```python
from build123d import *

# Parameters (mm, degrees)
BOSS_EXTRUDE1_DEPTH = 14
SKETCH2_R           = 2
CUT_EXTRUDE1_DEPTH  = 52.751714947


with BuildPart() as part:
    # Sketch1 → Boss-Extrude1 (new body)
    with BuildSketch(Plane.XY):
        with BuildLine():
            Line((0, 0), (42, 0))
            Line((42, 0), (42, 6))
            Line((42, 6), (30, 6))
            Line((30, 6), (30, 32.8))
            Line((30, 32.8), (22.249007882, 32.8))
            Line((22.249007882, 32.8), (22.249007882, 23.8))
            ThreePointArc((22.249007882, 23.8), (21, 15.999997414), (19.750992118, 23.8))
            Line((19.750992118, 23.8), (19.750992118, 32.8))
            Line((19.750992118, 32.8), (12, 32.8))
            Line((12, 32.8), (12, 6))
            Line((12, 6), (0, 6))
            Line((0, 6), (0, 0))
        make_face()
    extrude(amount=BOSS_EXTRUDE1_DEPTH)

    # Sketch2 → Cut-Extrude1 (cut, through all)
    with BuildSketch(Plane(origin=(0, 6, 0), x_dir=(1, 0, 0), z_dir=(0, 1, 0))):
        with Locations(Location((6, -7, 0), (0, 0, 180))):
            Circle(SKETCH2_R)
        with Locations(Location((36, -7, 0), (0, 0, 180))):
            Circle(SKETCH2_R)
    extrude(amount=-CUT_EXTRUDE1_DEPTH, mode=Mode.SUBTRACT)


solid = part.part
```
Design review of the part built by this model. Coordinates are the model's own, in mm. A direction names the side the tool comes from. Give positions to 0.01 mm unless a question says otherwise; leave off trailing zeros. Write each loop counter-clockwise with the first axis right and the second up, starting at its lowest first coordinate (ties: lowest second). Pieces come first, ordered by that corner, then holes. Notation, with made-up numbers: (52, -16) -> (72, -16) arc R20 cw to (72, 11) -> close; hole circle Ø11 at (-7, -7). An arc over 180 degrees is marked (long way). Answer in a Markdown table with one row per item.
(1) Consider section A-A (y = 29.5). State the section outline as (x, z) points, then the cut area to 3 significant figures.
Results:
| item | result |
|---|---|
| outline | (12, 0) -> (19.75, 0) -> (19.75, 14) -> (12, 14) -> close; (22.25, 0) -> (30, 0) -> (30, 14) -> (22.25, 14) -> close |
| area | 217 mm2 |
(2) Consider section C-C (x = 6). State the section outline as (y, z) points, then the cut area to 3 significant figures.
Results:
| item | result |
|---|---|
| outline | (0, 0) -> (6, 0) -> (6, 5) -> (0, 5) -> close; (0, 9) -> (6, 9) -> (6, 14) -> (0, 14) -> close |
| area | 60.0 mm2 |
(3) To check wall thickness, follow probe 1 along X at (y, z) = (20, 8.25); probe 2 along Z at (x, y) = (36, 1.85); probe 3 along X at (y, z) = (24, 6.5). State the ranges of each line that lie inside material, in increasing order.
Results:
| item | result |
|---|---|
| probe 1 | 12 to 17, 25 to 30 |
| probe 2 | 0 to 5, 9 to 14 |
| probe 3 | 12 to 19.75, 22.25 to 30 |
(4) Clearance check with flat-ended pins moving along their axes: pin 1 (9 mm diameter, centred on x = 21, y = 20, fed in from +Z); pin 2 (4.5 mm diameter, centred on y = 28, z = 8, fed in from +X); pin 3 (7 mm diameter, centred on y = 30, z = 7.5, fed in from -X); pin 4 (3 mm diameter, centred on x = 6, z = 7, fed in from +Y). State where each tip first meets the part, or that it passes through.
Results:
| item | result |
|---|---|
| pin 1 | z = 14 |
| pin 2 | x = 30 |
| pin 3 | x = 12 |
| pin 4 | through |
(5) Consider section B-B (z = 7). State the section outline as (x, y) points, then the cut area to 3 significant figures.
Results:
| item | result |
|---|---|
| outline | (0, 0) -> (4, 0) -> (4, 6) -> (0, 6) -> close; (8, 0) -> (34, 0) -> (34, 6) -> (30, 6) -> (30, 32.8) -> (22.25, 32.8) -> (22.25, 23.8) arc R4 cw (long way) to (19.75, 23.8) -> (19.75, 32.8) -> (12, 32.8) -> (12, 6) -> (8, 6) -> close; (38, 0) -> (42, 0) -> (42, 6) -> (38, 6) -> close |
| area | 614 mm2 |
(6) For faces 1 (the flat face through (0, 3, 7)), 2 (the flat face through (19.751, 28, 7)), 3 (the flat face through (7, 6, 5)), list the 3-axis set-ups (+Z, -Z, +X, -X, +Y, -Y) from which the entire face can be reached by the end or side of a thin tool; tool diameter is ignored.
Results:
| item | result |
|---|---|
| face 1 | +Z, -Z, -X, +Y, -Y |
| face 2 | +Z, -Z, +Y |
| face 3 | +Z, -Z, -X, +Y |
(7) Consider section D-D (z = 12). State the section outline as (x, y) points.
Results:
| item | result |
|---|---|
| outline | (0, 0) -> (42, 0) -> (42, 6) -> (30, 6) -> (30, 32.8) -> (22.25, 32.8) -> (22.25, 23.8) arc R4 cw (long way) to (19.75, 23.8) -> (19.75, 32.8) -> (12, 32.8) -> (12, 6) -> (0, 6) -> close |
(8) Mouldability with a two-part tool opening along X and no side actions: class faces 4 (the flat face through (12, 20, 7)), 5 (the cylindrical face through (7.474, 3.042, 8.352)), 6 (the flat face through (30, 19, 7)), 7 (the flat face through (37, 6, 5)) as +X half, -X half, draft (parallel to the pull), parting line (faces both ways), or undercut.
Results:
| item | result |
|---|---|
| face 4 | -X half |
| face 5 | undercut |
| face 6 | +X half |
| face 7 | draft |
